```python
from build123d import *

# Parameters (mm, degrees)
SKETCH1_W           = 182.149999994
SKETCH1_H           = 196.85
BOSS_EXTRUDE1_DEPTH = 12.7
FILLET1_R           = 12.7
HOLE1_D             = 3.175
HOLE1_DEPTH         = 31.75
HOLE1_CSINK_D       = 10.16
HOLE1_CSINK_ANGLE   = 82
HOLE1_TIP           = 0.953866233


with BuildPart() as part:
    # Sketch1 → Boss-Extrude1 (new body)
    with BuildSketch(Plane.XY):
        with Locations((47.975000003, 766.50216301)):
            Rectangle(SKETCH1_W, SKETCH1_H)
    extrude(amount=BOSS_EXTRUDE1_DEPTH)

    # Fillet1
    fillet1_edges = [part.edges().sort_by_distance(p)[0] for p in [
        (-43.099999994, 668.07716301, 6.35),
        (-43.099999994, 864.92716301, 6.35),
        (139.05, 864.92716301, 6.35),
        (139.05, 668.07716301, 6.35),
    ]]
    fillet(fillet1_edges, radius=FILLET1_R)

    # Hole1
    with Locations(Plane(origin=(47.975000003, -457.960607328, 12.7), x_dir=(1, 0, 0), z_dir=(0, 0, 1))):
        with Locations((-78.374999997, 1310.187770337), (-78.374999997, 1138.737770337), (78.374999997, 1138.737770337), (78.374999997, 1310.187770337)):
            CounterSinkHole(HOLE1_D / 2, HOLE1_CSINK_D / 2, depth=HOLE1_DEPTH, counter_sink_angle=HOLE1_CSINK_ANGLE)
            with Locations((0, 0, -(HOLE1_DEPTH + HOLE1_TIP / 2))):  # 118° drill point
                Cone(0, HOLE1_D / 2, HOLE1_TIP, mode=Mode.SUBTRACT)


solid = part.part
```
The model under review builds one solid part; all positions refer to its coordinate system, in mm. Round coordinates to 2 decimals unless told otherwise and drop trailing zeros. One line per question, with ' | ' between items.
Item 1: The part is to be moulded in two halves that separate along Y. For faces 1 (the face through (47, 768, 0)), 2 (the face through (126.73, 850.51, 8.88)), 3 (the face through (135.428, 861.108, 6.439)), 4 (the face through (-39.48, 671.9, 6.44)), say which applies: pulls with the +Y half, pulls with the -Y half, needs draft (parallel to the pull), parting line crosses it, or undercut.
Resolved:
face 1: needs draft | face 2: undercut | face 3: pulls with the +Y half | face 4: pulls with the -Y half
Item 2: To check wall thickness, follow probe 1 along Y at (x, z) = (125, 6.25); probe 2 along X at (y, z) = (855.5, 7.5); probe 3 along X at (y, z) = (854, 4.75). State the ranges of each line that lie inside material, in increasing order.
Resolved:
probe 1: y = 668.08 to 679.94, 681.61 to 851.39, 853.06 to 864.93 | probe 2: x = -42.67 to 138.62 | probe 3: x = -42.98 to 138.93
Item 3: For P1, Ø3.5, axis at x = 126.35, y = 680.78, coming from the +Z side; P2, Ø3, axis at x = -30.4, y = 680.78, coming from the -Z side; P3, Ø4, axis at x = 126.35, y = 852.23, coming from the +Z side, all flat-tipped, find the tip position at first contact; note any pin that passes through.
Resolved:
P1: stops at z = 8.87 | P2: passes through | P3: stops at z = 9.16
